For this review, take the finished solid that the model builds, in its own axes (mm). A direction names the side the tool comes from. Coordinates: 2 decimals unless noted, no trailing zeros. Loops run counter-clockwise (first coordinate to the right, second up) from the corner with the lowest first, then second, coordinate; pieces in that order, holes last.
1. Machinability: for faces 1 (the face through (-8.08, -23.87, -7.49)), 2 (the face through (35.56, -10, 34)), 3 (the face through (9.525, -10, -10)), 4 (the face through (8.08, -23.87, -6.48)), 5 (the face through (-23, -10, 24.13)), which of the approach directions +Z, -Z, +X, -X, +Y, -Y give a long, thin tool a straight path to every point of the face, cutting with its end or side? Answer none if there is none.
2. Take a section at D-D, the plane y = -23.5. State the section outline as (x, z) points.
3. Take a section at B-B, the plane z = -1.5. State the section outline as (x, y) points (3 decimals), then the cut area to 3 significant figures.
4. Take a section at A-A, the plane y = -7.25. State the section outline as (x, z) points (3 decimals), then the cut area to 3 significant figures.
5. Take a section at C-C, the plane x = 19. State the section outline as (y, z) points.
6. Clearance check with flat-ended pins moving along their axes: P1, Ø6, axis at x = 14, z = 20.5, coming from the +Y side; P2, Ø10, axis at x = 19.5, y = -10.5, coming from the -Z side; P3, Ø6, axis at y = -13.5, z = 2.5, coming from the +X side (3 decimals); P4, Ø10, axis at y = -8, z = 1.5, coming from the -X side (3 decimals). State where each tip first meets the part, or that it passes through.
7. To check wall thickness, follow probe 1 along Z at (x, y) = (11.5, -5.5); probe 2 along X at (y, z) = (-6.5, -28) (3 decimals); probe 3 along Y at (x, z) = (1, 38.5). State the ranges of each line that lie inside material, in increasing order.
```python
from build123d import *

# Parameters (mm, degrees)
F1_DEPTH = 25.4
F2_R     = 5.08


with BuildPart() as f1:
    # F0 (on Front) → F1 (new body)
    with BuildSketch(Plane.XZ):
        Polygon((-35.56, 43.18), (-35.56, 24.13), (-9.525, 24.13), (-9.525, -43.18), (9.525, -43.18), (9.525, 24.13), (35.56, 24.13), (35.56, 43.18), align=None)
    extrude(amount=F1_DEPTH)

    # F2
    f2_edges = [f1.edges().sort_by_distance(p)[0] for p in [
        (0, -25.4, 43.18),
        (35.56, -25.4, 33.655),
        (22.5425, -25.4, 24.13),
        (9.525, -25.4, -9.525),
        (0, -25.4, -43.18),
        (-9.525, -25.4, -9.525),
        (-22.5425, -25.4, 24.13),
        (-35.56, -25.4, 33.655),
    ]]
    fillet(f2_edges, radius=F2_R)


solid = f1.part
```
Results list:
1. face 1: -Z, -X, -Y
1. face 2: +Z, -Z, +X, +Y, -Y
1. face 3: -Z, +X, +Y, -Y
1. face 4: -Z, +X, -Y
1. face 5: -Z, -X, +Y, -Y
2. outline: (-34.44, 25.25) - (-8.41, 25.25) - (-8.41, -42.06) - (8.41, -42.06) - (8.41, 25.25) - (34.44, 25.25) - (34.44, 42.06) - (-34.44, 42.06) - close
3. outline: (-9.525, -20.32) arc R5.08 ccw to (-4.445, -25.4) - (4.445, -25.4) arc R5.08 ccw to (9.525, -20.32) - (9.525, 0) - (-9.525, 0) - close
3. area: 473 mm2
4. outline: (-35.56, 24.13) - (-9.525, 24.13) - (-9.525, -43.18) - (9.525, -43.18) - (9.525, 24.13) - (35.56, 24.13) - (35.56, 43.18) - (-35.56, 43.18) - close
4. area: 2,640 mm2
5. outline: (-25.4, 29.21) arc R5.08 ccw to (-20.32, 24.13) - (0, 24.13) - (0, 43.18) - (-20.32, 43.18) arc R5.08 ccw to (-25.4, 38.1) - close
6. P1: passes through
6. P2: stops at z = 24.13
6. P3: stops at x = 9.525
6. P4: stops at x = -9.525
7. probe 1: z = 24.13 to 43.18
7. probe 2: x = -9.525 to 9.525
7. probe 3: y = -25.38 to 0
